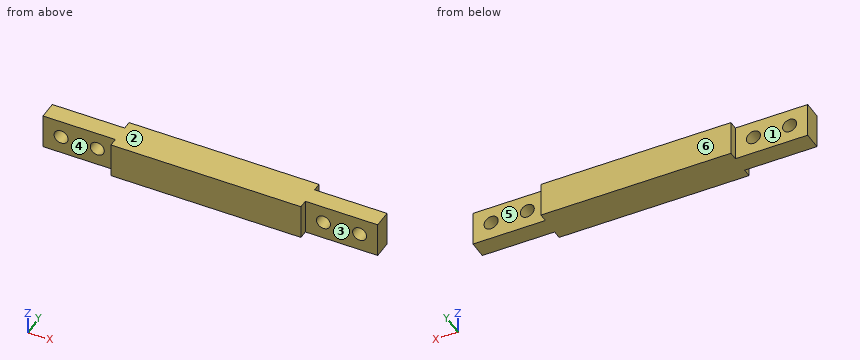
from build123d import *

# Parameters (mm, degrees)
PAD_DEPTH       = 7.8
SKETCH001_R     = 1.55
POCKET_DEPTH    = 5.901
POCKET001_DEPTH = 5.901


with BuildPart() as part:
    # Sketch → Pad (new body)
    with BuildSketch(Plane.XY):
        Polygon((37, -2), (37, 2), (21, 2), (21, 3.9), (-21, 3.9), (-21, 2), (-37, 2), (-37, -2), (-21, -2), (-21, -3.9), (21, -3.9), (21, -2), align=None)
    extrude(amount=PAD_DEPTH)

    # Sketch001 (on Face3 of Pad) → Pocket (cut, through all)
    with BuildSketch(Plane.XZ.offset(2)):
        with Locations((-33, 3.95)):
            Circle(SKETCH001_R)
        with Locations((-25, 3.95)):
            Circle(SKETCH001_R)
        with Locations((25, 3.95)):
            Circle(SKETCH001_R)
        with Locations((33, 3.95)):
            Circle(SKETCH001_R)
    extrude(amount=-POCKET_DEPTH, mode=Mode.SUBTRACT)

    # Sketch001 (on Face3 of Pad) → Pocket001 (cut, through all)
    with BuildSketch(Plane.XZ.offset(2)):
        with Locations((-33, 3.95)):
            Circle(SKETCH001_R)
        with Locations((-25, 3.95)):
            Circle(SKETCH001_R)
        with Locations((25, 3.95)):
            Circle(SKETCH001_R)
        with Locations((33, 3.95)):
            Circle(SKETCH001_R)
    extrude(amount=-POCKET001_DEPTH, mode=Mode.SUBTRACT)


solid = part.part
Work out the finished part from the listing and answer in its coordinate system (mm). Face numbers are marked on the shaded views. A direction names the side the tool comes from. Give positions to 0.01 mm unless a question says otherwise; leave off trailing zeros. Write each loop counter-clockwise with the first axis right and the second up, starting at its lowest first coordinate (ties: lowest second). Pieces come first, ordered by that corner, then holes.
Q1. The part is cut by section A-A on z = 3.95. Give the vertices of the cut face in (x, y), and give its area (3 significant figures).
Answer:
outline: (-37, -2) - (-34.55, -2) - (-34.55, 2) - (-37, 2) - close; (-31.45, -2) - (-26.55, -2) - (-26.55, 2) - (-31.45, 2) - close; (-23.45, -2) - (-21, -2) - (-21, -3.9) - (21, -3.9) - (21, -2) - (23.45, -2) - (23.45, 2) - (21, 2) - (21, 3.9) - (-21, 3.9) - (-21, 2) - (-23.45, 2) - close; (26.55, -2) - (31.45, -2) - (31.45, 2) - (26.55, 2) - close; (34.55, -2) - (37, -2) - (37, 2) - (34.55, 2) - close
area: 406 mm2
Q2. For a pull along Y with two mould halves and no side action, classify the marked faces 1, 2 and 3 as released by +Y, released by -Y, zero draft, split by the parting line, or undercut.
Answer:
face 1: released by +Y
face 2: zero draft
face 3: released by -Y
Q3. Given pin 1 (1 mm diameter, centred on y = -3, z = 3, fed in from +X); pin 2 (4 mm diameter, centred on x = 31, z = 5.5, fed in from +Y); pin 3 (1.5 mm diameter, centred on y = -3.5, z = 5, fed in from -X); pin 4 (3 mm diameter, centred on x = 25, z = 3.95, fed in from +Y), each flat-ended and moving along its own axis, determine where each tip first touches the part or whether it passes through.
Answer:
pin 1: stops at x = 21
pin 2: stops at y = 2
pin 3: stops at x = -21
pin 4: passes through
Q4. The part is cut by section B-B on x = 25. Give the vertices of the cut face in (y, z), and give its area (3 significant figures).
Answer:
outline: (-2, 0) - (2, 0) - (2, 2.4) - (-2, 2.4) - close; (-2, 5.5) - (2, 5.5) - (2, 7.8) - (-2, 7.8) - close
area: 18.8 mm2
Q5. Straight lines are drawn through the part: L1, parallel to Z at x = -33, y = 1; L2, parallel to X at y = -2.25, z = 6.75; L3, parallel to Y at x = -22.5, z = 1. For each, find the intervals that lie inside material, in ascending order.
Answer:
L1: z = 0 to 2.4, 5.5 to 7.8
L2: x = -21 to 21
L3: y = -2 to 2
Q6. The part is cut by section D-D on y = 3.25. Give the vertices of the cut face in (x, z), and give its area (3 significant figures).
Answer:
outline: (-21, 0) - (21, 0) - (21, 7.8) - (-21, 7.8) - close
area: 328 mm2
Q7. The part is cut by section C-C on x = -29. Give the vertices of the cut face in (y, z), and give its area (3 significant figures).
Answer:
outline: (-2, 0) - (2, 0) - (2, 7.8) - (-2, 7.8) - close
area: 31.2 mm2
Q8. A tool of negligible diameter and unlimited length cuts with its end or side. For the marked faces 4, 5 and 6, from which of +Z, -Z, +X, -X, +Y, -Y can it reach the whole face along a straight path? Write none if from no direction.
Answer:
face 4: +Z, -Z, -X, -Y
face 5: +Z, -Z, +X, +Y
face 6: +Z, -Z, +X, -X, +Y
